Design review of the part built by this model. Coordinates are the model's own, in mm. Coordinates: 2 decimals unless noted, no trailing zeros. Loops run counter-clockwise (first coordinate to the right, second up) from the corner with the lowest first, then second, coordinate; pieces in that order, holes last. Notation, with made-up numbers: (29.5, 17) -> (76.5, 17) arc R23 ccw to (76.5, 34) -> close; hole circle Ø4 at (59, 66.25). An arc over 180 degrees is marked (long way). Use a Markdown table: item, result. Add a question column.
Q1. Take a section at A-A on y = 0. Count the separate pieces of the cut face and the enclosed holes in it, plus the area to 3 significant figures.
Q2. For probe 1 along Y at (x, z) = (1, 60); probe 2 along Z at (x, y) = (0, 4.6), list the stretches that pass through material, from the lowest coordinate up.
Q3. Take a section at B-B on z = 51. Write out the cut boundary in (x, y), plus the area to 3 significant figures.
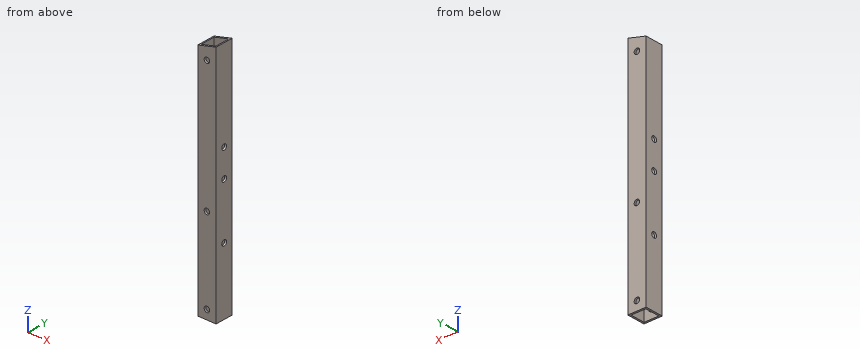
from build123d import *

# Parameters (mm, degrees)
SKETCH_1_W          = 10
SKETCH_1_H          = 10
SKETCH_1_W_2        = 8
SKETCH_1_H_2        = 8
EXTRUDE_1_DEPTH     = 130
SKETCH_2_R          = 1.5
CUT_EXTRUDE_1_DEPTH = 11
SKETCH_3_R          = 1.5
CUT_EXTRUDE_2_DEPTH = 11


with BuildPart() as part:
    # 草图1 → 拉伸-薄壁1 (new body)
    with BuildSketch(Plane.XY):
        Rectangle(SKETCH_1_W, SKETCH_1_H)
        Rectangle(SKETCH_1_W_2, SKETCH_1_H_2, mode=Mode.SUBTRACT)
    extrude(amount=EXTRUDE_1_DEPTH)

    # 草图2 → 切除-拉伸1 (cut, through all)
    with BuildSketch(Plane.XZ.offset(5)):
        with Locations((0, 51)):
            Circle(SKETCH_2_R)
        with Locations((0, 122)):
            Circle(SKETCH_2_R)
        with Locations((0, 5)):
            Circle(SKETCH_2_R)
        Polygon((5, 130), (-5, 127.320508076), (-5, 130), align=None)
    extrude(amount=-CUT_EXTRUDE_1_DEPTH, mode=Mode.SUBTRACT)

    # 草图3 → 切除-拉伸2 (cut, through all)
    with BuildSketch(Plane(origin=(5, 0, 0), x_dir=(0, 0, -1), z_dir=(1, 0, 0))):
        with Locations((-36, 0)):
            Circle(SKETCH_3_R)
        with Locations((-66, 0)):
            Circle(SKETCH_3_R)
        with Locations((-81, 0)):
            Circle(SKETCH_3_R)
    extrude(amount=-CUT_EXTRUDE_2_DEPTH, mode=Mode.SUBTRACT)


solid = part.part
Answer list:
| question | item | result |
|---|---|---|
| 1 | separate pieces | 8 |
| 1 | enclosed holes | 0 |
| 1 | area | 239 mm² |
| 2 | probe 1 | -5 to -4, 4 to 5 |
| 2 | probe 2 | 0 to 3.5, 6.5 to 49.5, 52.5 to 120.5, 123.5 to 128.66 |
| 3 | outline | (-5, -5) -> (-1.5, -5) -> (-1.5, -4) -> (-4, -4) -> (-4, 4) -> (-1.5, 4) -> (-1.5, 5) -> (-5, 5) -> close; (1.5, -5) -> (5, -5) -> (5, 5) -> (1.5, 5) -> (1.5, 4) -> (4, 4) -> (4, -4) -> (1.5, -4) -> close |
| 3 | area | 30.0 mm² |
